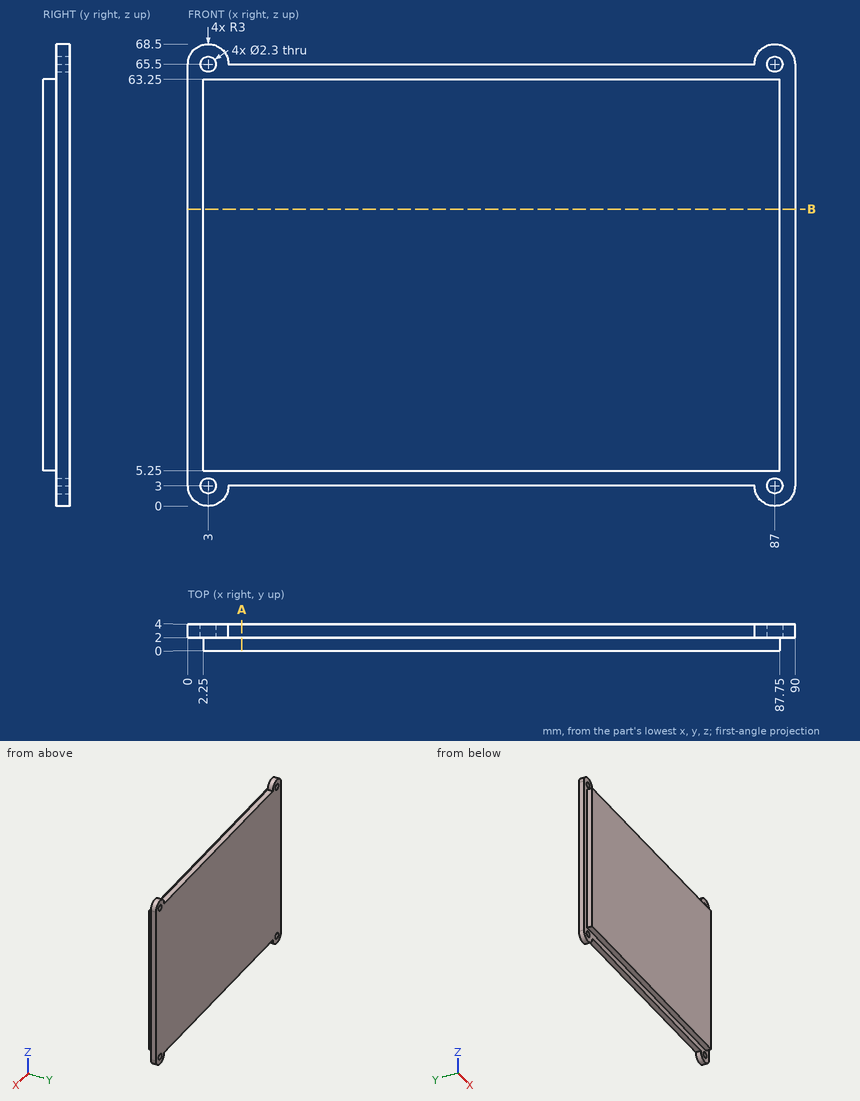
Geometry check sheet. Reference: drawing and pictorial views, mm from the part's lowest x, y, z. Give positions to 0.01 mm unless a question says otherwise; leave off trailing zeros. Loops run counter-clockwise (first coordinate to the right, second up) from the corner with the lowest first, then second, coordinate; pieces in that order, holes last.
1. Section check B-B, the plane z = 44. Enter the section's corners in (x, y).
2. Thickness scan on line 1 (Z direction, x = 87, y = 3.55); line 2 (Z direction, x = 29.5, y = 1.3); line 3 (Y direction, x = 4, z = 63.5). Record the ranges inside material, lowest first.
3. Section check A-A, the plane x = 8. Enter the section's corners in (y, z), then the cut area to 3 significant figures.
4. Go/stop test with flat-tipped pins: pin 1 Ø1 at (x, y) = (57.5, 3) entering from +Z; pin 2 Ø1.6 at (x, y) = (47, 1) entering from -Z; pin 3 Ø1.4 at (x, z) = (87, 3) entering from -Y; pin 4 Ø1 at (x, y) = (43.5, 2.5) entering from -Z. Record where each tip stops, or that it passes through.
Geometry says:
1. outline: (0, 2) - (2.25, 2) - (2.25, 0) - (87.75, 0) - (87.75, 2) - (90, 2) - (90, 4) - (0, 4) - close
2. line 1: z = 0 to 1.85, 4.15 to 64.35, 66.65 to 68.5
2. line 2: z = 5.25 to 63.25
2. line 3: y = 2 to 4
3. outline: (0, 5.25) - (2, 5.25) - (2, 3) - (4, 3) - (4, 65.5) - (2, 65.5) - (2, 63.25) - (0, 63.25) - close
3. area: 241 mm2
4. pin 1: stops at z = 65.5
4. pin 2: stops at z = 5.25
4. pin 3: passes through
4. pin 4: stops at z = 3
